from build123d import *

# Parameters (mm, degrees)
PAD_DEPTH    = 1
PAD001_DEPTH = 28.1
PAD002_DEPTH = 1
SKETCH003_R  = 0.6
POCKET_DEPTH = 30.1


with BuildPart() as part:
    # Sketch → Pad (new body)
    with BuildSketch(Plane.XY):
        Polygon((0, 0), (60, 0), (60, 0.5), (30, 25.5), (0, 0.5), align=None)
    extrude(amount=PAD_DEPTH)

    # Sketch001 (on Face7 of Pad) → Pad001 (join)
    with BuildSketch(Plane.XY.offset(1)):
        Polygon((0, 0), (0, 0.5), (23.756329, 2.5), (30, 25.5), (36.243671, 2.5), (60, 0.5), (60, 0), align=None)
    extrude(amount=PAD001_DEPTH)

    # Sketch002 (on Face13 of Pad001) → Pad002 (join)
    with BuildSketch(Plane.XY.offset(29.1)):
        Polygon((0, 0), (0, 0.5), (30, 25.5), (60, 0.5), (60, 0), align=None)
    extrude(amount=PAD002_DEPTH)

    # Sketch003 (on Face20 of Pad002) → Pocket (cut)
    with BuildSketch(Plane.XY.offset(30.1)):
        with Locations((30, 2.5)):
            Circle(SKETCH003_R)
    extrude(amount=-POCKET_DEPTH, mode=Mode.SUBTRACT)


solid = part.part
Geometry check sheet. Reference: the model listing, model coordinates, mm. A direction names the side the tool comes from. Give positions to 0.01 mm unless a question says otherwise; leave off trailing zeros. Loops run counter-clockwise (first coordinate to the right, second up) from the corner with the lowest first, then second, coordinate; pieces in that order, holes last.
(1) Section check A-A on z = 26. Record the cut outline in (x, y).
From the geometry:
outline: (0, 0) - (60, 0) - (60, 0.5) - (36.24, 2.5) - (30, 25.5) - (23.76, 2.5) - (0, 0.5) - close; hole circle Ø1.2 at (30, 2.5)
(2) Section check D-D on y = 21.5. Record the cut outline in (x, z), then the cut area to 3 significant figures.
From the geometry:
outline: (25.2, 0) - (34.8, 0) - (34.8, 1) - (31.09, 1) - (31.09, 29.1) - (34.8, 29.1) - (34.8, 30.1) - (25.2, 30.1) - (25.2, 29.1) - (28.91, 29.1) - (28.91, 1) - (25.2, 1) - close
area: 80.2 mm2
(3) Section check C-C on x = 27. Record the cut outline in (y, z).
From the geometry:
outline: (0, 0) - (23, 0) - (23, 1) - (14.45, 1) - (14.45, 29.1) - (23, 29.1) - (23, 30.1) - (0, 30.1) - close
(4) Release check for a two-part mould opening along Z. For faces 1 (the flat face through (18, 9, 1)), 2 (the flat face through (30, 10, 30.1)), 3 (the flat face through (14.79, 12.825, 29.593)) record: released by +Z, released by -Z, zero draft, split by the parting line, or undercut.
From the geometry:
face 1: undercut
face 2: released by +Z
face 3: zero draft
(5) Thickness scan on L1, parallel to Z at x = 16, y = 5; L2, parallel to X at y = 23.5, z = 9.5; L3, parallel to Y at x = 3.5, z = 6. Record the ranges inside material, lowest first.
From the geometry:
L1: z = 0 to 1, 29.1 to 30.1
L2: x = 29.46 to 30.54
L3: y = 0 to 0.79
(6) Section check B-B on y = 6. Record the cut outline in (x, z), then the cut area to 3 significant figures.
From the geometry:
outline: (6.6, 0) - (53.4, 0) - (53.4, 1) - (35.29, 1) - (35.29, 29.1) - (53.4, 29.1) - (53.4, 30.1) - (6.6, 30.1) - (6.6, 29.1) - (24.71, 29.1) - (24.71, 1) - (6.6, 1) - close
area: 391 mm2
(7) Depth check by flat-ended pin: pin 1 Ø8 at (y, z) = (15, 19.5) entering from +X; pin 2 Ø4 at (y, z) = (12.5, 23.5) entering from -X; pin 3 Ø7.5 at (x, y) = (11.5, 11) entering from -Z; pin 4 Ø1.5 at (y, z) = (14, 23) entering from -X. Enter the tip coordinate at first touch or a pass-through.
From the geometry:
pin 1: stops at x = 33.94
pin 2: stops at x = 25.93
pin 3: stops at z = 0
pin 4: stops at x = 26.67
(8) Set-up check for faces 4 (the flat face through (42, 9, 29.1)), 5 (the flat face through (11.712, 1.486, 14.853)), 6 (the flat face through (30, 0, 15)): record each of +Z, -Z, +X, -X, +Y, -Y from which the full face is reachable in a straight line by a thin tool's end or side.
From the geometry:
face 4: +X, +Y
face 5: -X, +Y
face 6: +Z, -Z, +X, -X, -Y
